Build history of the part. All positions in model axes, mm. Face numbers are marked on the shaded views. Round coordinates to 2 decimals unless told otherwise and drop trailing zeros. Order: outer loops, then holes, each group sorted by start corner. A loop starts at its lowest first (then second) coordinate and runs counter-clockwise, first axis right, second up. Notation, with made-up numbers: (58, 77.5) -> (109, 77.5) arc R21 ccw to (109, 82.5) -> close; hole circle Ø2 at (-16, 9.5). An arc over 180 degrees is marked (long way). Use a Markdown table: item, result. Add a question column.
Item 1: Two-plate mould, pull along Y, no slides. Class the marked faces 1, 2 and 3: released by +Y, released by -Y, zero draft, split by the parting line, or undercut.
Item 2: Slice it at B-B, the plane z = 0. Give the cut face in (x, y), plus the area to 3 significant figures.
Item 3: Slice it at A-A, the plane y = 42.5. Give the cut face in (x, z).
Item 4: Slice it at C-C, the plane y = -24. Give the cut face in (x, z).
Item 5: Pin check, flat tips, straight feed: pin 1 (0.6 mm diameter, centred on y = 40.5, z = 40.5, fed in from -X); pin 2 (6 mm diameter, centred on x = -0.5, y = -16, fed in from -Z); pin 3 (1.2 mm diameter, centred on x = 4.5, y = 4, fed in from +Z). Stop position of each tip, or through.
Item 6: Probe L1, parallel to Y at x = 0, z = 40.55; L2, parallel to Y at x = 4.25, z = -1.5; L3, parallel to Y at x = 0, z = 39.5. List the from-to ranges inside material, lowest first.
from build123d import *

# Parameters (mm, degrees)
BOSS_EXTRUDE1_DEPTH   = 11
BOSS_EXTRUDE1_2_DEPTH = 11
SKETCH2_W             = 15.446473034
SKETCH2_H             = 16.677637278
BOSS_EXTRUDE2_DEPTH   = 4
SKETCH3_R             = 3
BOSS_EXTRUDE3_DEPTH   = 4
BOSS_EXTRUDE4_DEPTH   = 2.8
CUT_EXTRUDE1_DEPTH    = 11
SKETCH11_W            = 0.1
SKETCH11_H            = 16.677637278
CUT_EXTRUDE2_DEPTH    = 11
SKETCH12_W            = 8
SKETCH12_H            = 14
SKETCH12_R            = 1.6
BOSS_EXTRUDE5_DEPTH   = 3
FILLET1_R             = 1
SKETCH14_W            = 1.465452289
SKETCH14_H            = 3.319739537
SKETCH14_W_2          = 1.579669893
CUT_EXTRUDE3_DEPTH    = 3
SKETCH15_W            = 1.507141025
SKETCH15_H            = 3.716681852
SKETCH15_W_2          = 1.554838049
SKETCH15_H_2          = 3.443775751
CUT_EXTRUDE4_DEPTH    = 3


with BuildPart() as part:
    # Sketch1 → Boss-Extrude1 (new body)
    with BuildSketch(Plane(origin=(0, 0, 0), x_dir=(1, 0, 0), z_dir=(0, 1, 0))):
        Polygon((6.574205289, -3.388868816), (7.883511398, -3.388868816), (7.883511398, -9.402687455), (-7.562961636, -9.402687455), (-7.562961636, -3.388868816), (-6.253655527, -3.388868816), (-5.025255986, -6.763868816), (-4.078972201, -6.763868816), (-2.850572661, -3.388868816), (-1.541266552, -3.388868816), (-0.312867011, -6.763868816), (0.633416774, -6.763868816), (1.861816314, -3.388868816), (3.171122423, -3.388868816), (4.399521964, -6.763868816), (5.345805749, -6.763868816), align=None)
    extrude(amount=BOSS_EXTRUDE1_DEPTH)



with BuildPart() as body_2:
    # Sketch1 → Boss-Extrude1 2 (new body)
    with BuildSketch(Plane(origin=(0, 0, 0), x_dir=(1, 0, 0), z_dir=(0, 1, 0))):
        Polygon((6.574205289, 1.261131184), (7.883511398, 1.261131184), (7.883511398, 7.274949823), (-7.562961636, 7.274949823), (-7.562961636, 1.261131184), (-6.253655527, 1.261131184), (-5.025255986, 4.636131184), (-4.078972201, 4.636131184), (-2.850572661, 1.261131184), (-1.541266552, 1.261131184), (-0.312867011, 4.636131184), (0.633416774, 4.636131184), (1.861816314, 1.261131184), (3.171122423, 1.261131184), (4.399521964, 4.636131184), (5.345805749, 4.636131184), align=None)
    extrude(amount=BOSS_EXTRUDE1_2_DEPTH)


with BuildPart() as part_1:
    add(part.part)

    add(body_2.part)  # Boss-Extrude2 merges body 2
    # Sketch2 → Boss-Extrude2 (add)
    with BuildSketch(Plane(origin=(0, 11, 0), x_dir=(1, 0, 0), z_dir=(0, 1, 0))):
        with Locations((0.160274881, -1.063868816)):
            Rectangle(SKETCH2_W, SKETCH2_H)
    extrude(amount=BOSS_EXTRUDE2_DEPTH)

    # Sketch3 → Boss-Extrude3 (add)
    with BuildSketch(Plane.XY.offset(9.402687455)):
        with Locations((0.160274881, 7.5)):
            Circle(SKETCH3_R)
    extrude(amount=BOSS_EXTRUDE3_DEPTH)

    # Sketch7 → Boss-Extrude4 (add, symmetric)
    with BuildSketch(Plane(origin=(0, 0, 0), x_dir=(0, 0, -1), z_dir=(1, 0, 0))):
        with BuildLine():
            Line((-41.402687455, -22.5), (-41.402687455, -18.5))
            ThreePointArc((-41.402687455, -18.5), (-15.402687455, 7.5), (-41.402687455, 33.5))
            Line((-41.402687455, 33.5), (-41.402687455, 37.5))
            ThreePointArc((-41.402687455, 37.5), (-11.402687455, 7.5), (-41.402687455, -22.5))
        make_face()
    extrude(amount=BOSS_EXTRUDE4_DEPTH, both=True)

    # Sketch9 → Cut-Extrude1 (cut)
    with BuildSketch(Plane(origin=(0, 0, 0), x_dir=(-1, 0, 0), z_dir=(0, -1, 0))):
        Polygon((7.462961636, -9.402687455), (7.462961636, -3.488868816), (6.323676281, -3.488868816), (5.09527674, -6.863868816), (4.008951448, -6.863868816), (2.780551907, -3.488868816), (1.611287306, -3.488868816), (0.382887765, -6.863868816), (-0.703437527, -6.863868816), (-1.931837068, -3.488868816), (-3.101101669, -3.488868816), (-4.32950121, -6.863868816), (-5.415826502, -6.863868816), (-6.644226043, -3.488868816), (-7.783511398, -3.488868816), (-7.783511398, -9.402687455), (-7.883511398, -9.402687455), (-7.883511398, -3.388868816), (-6.574205289, -3.388868816), (-5.345805749, -6.763868816), (-4.399521964, -6.763868816), (-3.171122423, -3.388868816), (-1.861816314, -3.388868816), (-0.633416774, -6.763868816), (0.312867011, -6.763868816), (1.541266552, -3.388868816), (2.850572661, -3.388868816), (4.078972201, -6.763868816), (5.025255986, -6.763868816), (6.253655527, -3.388868816), (7.562961636, -3.388868816), (7.562961636, -9.402687455), align=None)
        Polygon((7.562961636, 1.261131184), (7.562961636, 7.274949823), (7.462961636, 7.274949823), (7.462961636, 1.361131184), (6.323676281, 1.361131184), (5.09527674, 4.736131184), (4.008951448, 4.736131184), (2.780551907, 1.361131184), (1.611287306, 1.361131184), (0.382887765, 4.736131184), (-0.703437527, 4.736131184), (-1.931837068, 1.361131184), (-3.101101669, 1.361131184), (-4.32950121, 4.736131184), (-5.415826502, 4.736131184), (-6.644226043, 1.361131184), (-7.783511398, 1.361131184), (-7.783511398, 7.274949823), (-7.883511398, 7.274949823), (-7.883511398, 1.261131184), (-6.574205289, 1.261131184), (-5.345805749, 4.636131184), (-4.399521964, 4.636131184), (-3.171122423, 1.261131184), (-1.861816314, 1.261131184), (-0.633416774, 4.636131184), (0.312867011, 4.636131184), (1.541266552, 1.261131184), (2.850572661, 1.261131184), (4.078972201, 4.636131184), (5.025255986, 4.636131184), (6.253655527, 1.261131184), align=None)
    extrude(amount=-CUT_EXTRUDE1_DEPTH, mode=Mode.SUBTRACT)

    # Sketch11 → Cut-Extrude2 (cut)
    with BuildSketch(Plane.XZ.offset(-11)):
        with Locations((7.833511398, 1.063868816)):
            Rectangle(SKETCH11_W, SKETCH11_H)
        with Locations((-7.512961636, 1.063868816)):
            Rectangle(SKETCH11_W, SKETCH11_H)
    extrude(amount=-CUT_EXTRUDE2_DEPTH, mode=Mode.SUBTRACT)

    # Sketch12 → Boss-Extrude5 (add)
    with BuildSketch(Plane.XY.offset(41.402687455)):
        with Locations((0, -25.5)):
            Rectangle(SKETCH12_W, SKETCH12_H)
        with Locations((0, -27.5)):
            Circle(SKETCH12_R, mode=Mode.SUBTRACT)
    boss_extrude5 = extrude(amount=-BOSS_EXTRUDE5_DEPTH)

    # Mirror1: Boss-Extrude5 across plane
    add(boss_extrude5.mirror(Plane.ZX.offset(7.5)))

    # Fillet1
    fillet1_edges = [part_1.edges().sort_by_distance(p)[0] for p in [
        (0.160274881, 0, 9.402687455),
        (-7.462961636, 7.5, 9.402687455),
        (7.783511398, 7.5, 9.402687455),
        (-2.839725119, 7.5, 9.402687455),
        (-7.462961636, 7.5, -7.274949823),
        (0.160274881, 0, -7.274949823),
        (7.783511398, 7.5, -7.274949823),
        (0.160274881, 15, 9.402687455),
        (-7.462961636, 15, 1.063868816),
        (0.160274881, 15, -7.274949823),
        (7.783511398, 15, 1.063868816),
        (0, -32.5, 38.402687455),
        (-4, -25.5, 38.402687455),
        (4, -25.5, 38.402687455),
        (0, 47.5, 38.402687455),
        (4, 40.5, 38.402687455),
        (-4, 40.5, 38.402687455),
        (-2.8, 27.804389345, 19.318037281),
        (2.8, 28.147641568, 19.638613901),
        (-2.8, -12.804389345, 19.318037281),
        (2.8, -13.147641568, 19.638613901),
    ]]
    fillet(fillet1_edges, radius=FILLET1_R)

    # Sketch14 → Cut-Extrude3 (cut)
    with BuildSketch(Plane.XZ.offset(-33.5)):
        with Locations((-3.532726145, 39.742817687)):
            Rectangle(SKETCH14_W, SKETCH14_H)
        with Locations((3.589834946, 39.742817687)):
            Rectangle(SKETCH14_W_2, SKETCH14_H)
    extrude(amount=-CUT_EXTRUDE3_DEPTH, mode=Mode.SUBTRACT)

    # Sketch15 → Cut-Extrude4 (cut)
    with BuildSketch(Plane(origin=(0, -18.5, 0), x_dir=(1, 0, 0), z_dir=(0, 1, 0))):
        with Locations((3.553570513, -39.544346529)):
            Rectangle(SKETCH15_W, SKETCH15_H)
        with Locations((-3.577419025, -39.68079958)):
            Rectangle(SKETCH15_W_2, SKETCH15_H_2)
    extrude(amount=-CUT_EXTRUDE4_DEPTH, mode=Mode.SUBTRACT)


solid = part_1.part
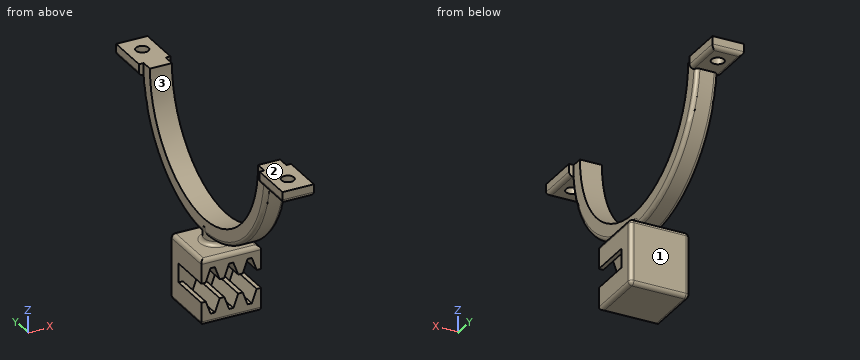
Check sheet entries:
| question | item | result |
|---|---|---|
| 1 | face 1 | released by +Y |
| 1 | face 2 | zero draft |
| 1 | face 3 | undercut |
| 2 | outline | (-7.46, 11) -> (7.78, 11) -> (7.78, 14) arc R1 ccw to (6.78, 15) -> (-6.46, 15) arc R1 ccw to (-7.46, 14) -> close |
| 2 | area | 60.6 mm2 |
| 3 | outline | (-4, 39.4) arc R1 ccw to (-3, 38.4) -> (-1.6, 38.4) -> (-1.6, 41.4) -> (-4, 41.4) -> close; (1.6, 38.4) -> (3, 38.4) arc R1 ccw to (4, 39.4) -> (4, 41.4) -> (1.6, 41.4) -> close |
| 4 | outline | (-4, 39.4) arc R1 ccw to (-3, 38.4) -> (3, 38.4) arc R1 ccw to (4, 39.4) -> (4, 41.4) -> (-4, 41.4) -> close |
| 5 | pin 1 | x = -4 |
| 5 | pin 2 | z = 19.5 |
| 5 | pin 3 | z = 9.4 |
| 6 | L1 | -32.5 to -29.1, -25.9 to -18.49, 33.49 to 40.9, 44.1 to 47.5 |
| 6 | L2 | 11 to 15 |
| 6 | L3 | -32.5 to -29.1, -25.9 to -18.43, 33.43 to 40.9, 44.1 to 47.5 |
